Can you work these out from the drawing? Everything is in mm from the part's minimum corner. A direction names the side the tool comes from. Coordinates: 2 decimals unless noted, no trailing zeros. Order: outer loops, then holes, each group sorted by start corner. A loop starts at its lowest first (then second) coordinate and runs counter-clockwise, first axis right, second up. Notation, with made-up numbers: (0, 34) -> (15, 34) arc R20 cw to (15, 62) -> close; hole circle Ø6 at (-33, 85). An arc over 180 degrees is marked (long way). Return JSON: item names as keys, results as strings. Group by question number.
1) If we section it at D-D, the plane y = 16.5: Please give me the cut outline in (x, z).
2) If we section it at B-B, the plane x = 45: Please give me the cut outline in (y, z), then the cut area to 3 significant figures.
3) If I drill on probe 1 along Y at (x, z) = (33.5, 42.5); probe 2 along Y at (x, z) = (15.5, 24); probe 3 along X at (y, z) = (8, 7), over which ranges is the centre line in solid material (lowest first)? Write a range as from..to.
4) If we section it at A-A, the plane y = 12.5: Please give me the cut outline in (x, z), then the cut area to 4 significant figures.
5) For pin 1 (8 mm diameter, centred on x = 10, z = 29.5, fed in from -Y); pin 2 (2 mm diameter, centred on x = 61, y = 18.5, fed in from -Z); pin 3 (5 mm diameter, centred on x = 15, y = 20, fed in from +Z), each with a flat end and sliding along its axis, tell me the tip position at first contact or that it passes through.
6) For the marked faces 1, 2 and 3, which set-ups out of +Z, -Z, +X, -X, +Y, -Y let a thin tool reach every point of the face, with its end or its side?
7) If we section it at C-C, the plane z = 31: Please give me the cut outline in (x, y).
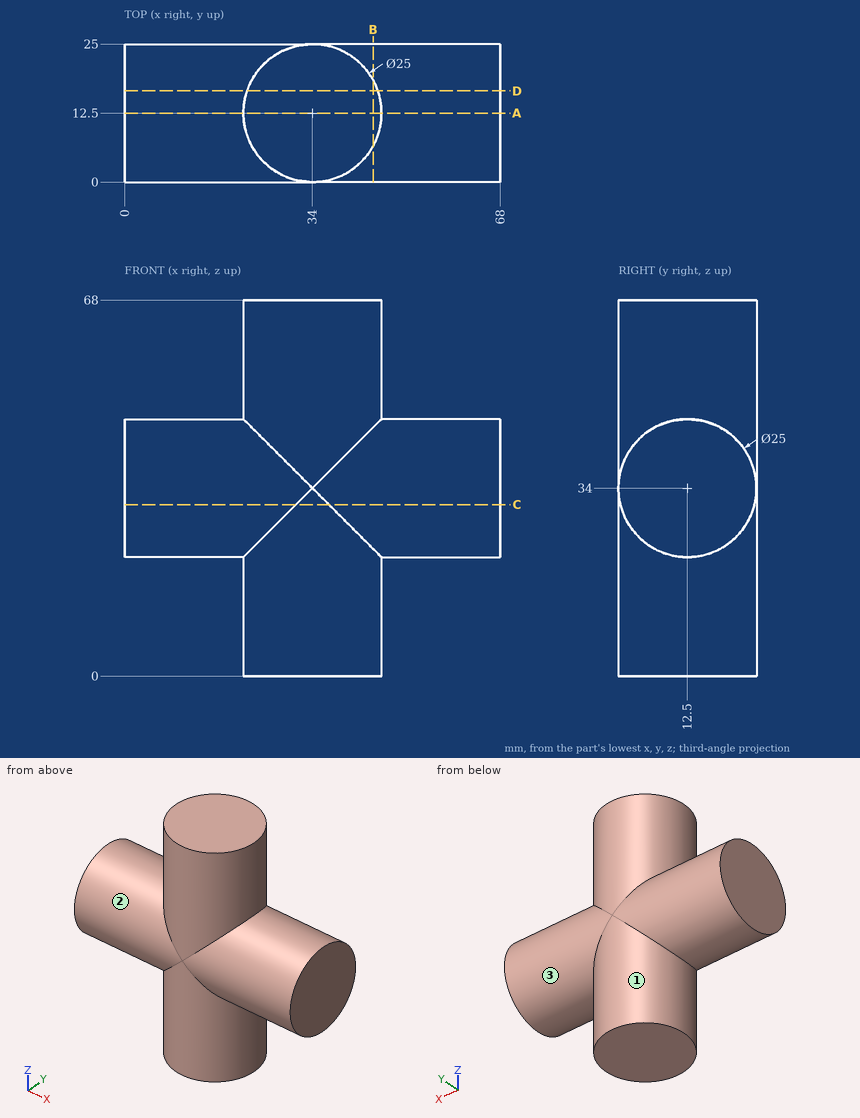
Result sheet:
{
 "1": {"outline": "(0, 22.16) -> (22.16, 22.16) -> (22.16, 0) -> (45.84, 0) -> (45.84, 22.16) -> (68, 22.16) -> (68, 45.84) -> (45.84, 45.84) -> (45.84, 68) -> (22.16, 68) -> (22.16, 45.84) -> (0, 45.84) -> close"},
 "2": {"outline": "(6.56, 0) -> (18.44, 0) -> (18.44, 23) arc R12.5 ccw to (18.44, 45) -> (18.44, 68) -> (6.56, 68) -> (6.56, 45) arc R12.5 ccw to (6.56, 23) -> close", "area": "1,010 mm2"},
 "3": {"probe 1": "y = 0.01..24.99", "probe 2": "y = 5..20", "probe 3": "x = 22.34..45.66"},
 "4": {"outline": "(0, 21.5) -> (21.5, 21.5) -> (21.5, 0) -> (46.5, 0) -> (46.5, 21.5) -> (68, 21.5) -> (68, 46.5) -> (46.5, 46.5) -> (46.5, 68) -> (21.5, 68) -> (21.5, 46.5) -> (0, 46.5) -> close", "area": "2,775 mm2"},
 "5": {"pin 1": "stops at y = 0.01", "pin 2": "stops at z = 22.54", "pin 3": "stops at z = 45.46"},
 "6": {"face 1": "-Z", "face 2": "-X", "face 3": "+X"},
 "7": {"outline": "(0, 0.37) -> (31, 0.37) arc R12.5 ccw to (37, 0.37) -> (68, 0.37) -> (68, 24.63) -> (37, 24.63) arc R12.5 ccw to (31, 24.63) -> (0, 24.63) -> close"}
}
